Source: CAD feature listing. Evaluate the final solid. Frame: model axes, mm. Face numbers are marked on the shaded views. Give positions to 0.01 mm unless a question says otherwise; leave off trailing zeros. Order: outer loops, then holes, each group sorted by start corner. A loop starts at its lowest first (then second) coordinate and runs counter-clockwise, first axis right, second up. Notation, with made-up numbers: (-9.75, 27.25) -> (20.25, 27.25) arc R10 ccw to (20.25, 41.25) -> close; hole circle Ø5 at (81, -15.5). An arc over 180 degrees is marked (long way). Answer in a Markdown table with one row per item.
```python
from build123d import *

# Parameters (mm, degrees)
SKETCH1_W           = 5.2324
SKETCH1_H           = 13.97
BOSS_EXTRUDE1_DEPTH = 1.524
BOSS_EXTRUDE2_DEPTH = 12.954
SKETCH3_W           = 1.1176
SKETCH3_H           = 1.524
BOSS_EXTRUDE3_DEPTH = 1.016
SKETCH4_W           = 3.81
SKETCH4_H           = 0.1651
BOSS_EXTRUDE4_DEPTH = 1.016
SKETCH5_W           = 3.81
SKETCH5_H           = 0.1651
BOSS_EXTRUDE5_DEPTH = 1.3589
SKETCH6_W           = 13.8049
SKETCH6_H           = 1.3589
CUT_EXTRUDE1_DEPTH  = 0.9525
SKETCH7_W           = 13.8049
SKETCH7_H           = 1.3589
CUT_EXTRUDE2_DEPTH  = 2.4384
SKETCH8_W           = 1.651
SKETCH8_H           = 0.381
CUT_EXTRUDE3_DEPTH  = 1.524
CUT_EXTRUDE4_DEPTH  = 10.995150124
CHAMFER1_SIZE       = 1.143
CHAMFER1_SIZE2      = 0.9906
CHAMFER2_SIZE       = 1.143
CHAMFER2_SIZE_2     = 0.9906


with BuildPart() as part:
    # Sketch1 → Boss-Extrude1 (new body)
    with BuildSketch(Plane(origin=(0, 1.524, 0), x_dir=(-1, 0, 0), z_dir=(0, 1, 0))):
        with Locations((-4.3688, 0)):
            Rectangle(SKETCH1_W, SKETCH1_H)
    extrude(amount=-BOSS_EXTRUDE1_DEPTH)

    # Sketch2 → Boss-Extrude2 (add)
    with BuildSketch(Plane.XY.offset(6.985)):
        Polygon((-5.8674, 1.3589), (1.7526, 1.3589), (1.7526, 1.524), (-6.985, 1.524), (-6.985, 0), (-5.8674, 0), align=None)
    extrude(amount=-BOSS_EXTRUDE2_DEPTH)

    # Sketch3 → Boss-Extrude3 (add)
    with BuildSketch(Plane(origin=(0, 0, -5.969), x_dir=(-1, 0, 0), z_dir=(0, 0, -1))):
        with Locations((6.4262, 0.762)):
            Rectangle(SKETCH3_W, SKETCH3_H)
    extrude(amount=BOSS_EXTRUDE3_DEPTH)

    # Sketch4 → Boss-Extrude4 (add)
    with BuildSketch(Plane(origin=(0, 0, -5.969), x_dir=(-1, 0, 0), z_dir=(0, 0, -1))):
        with Locations((2.0574, 1.44145)):
            Rectangle(SKETCH4_W, SKETCH4_H)
    extrude(amount=BOSS_EXTRUDE4_DEPTH)

    # Sketch5 → Boss-Extrude5 (add)
    with BuildSketch(Plane.XZ.offset(-1.3589)):
        with Locations((-2.0574, -6.90245)):
            Rectangle(SKETCH5_W, SKETCH5_H)
    extrude(amount=BOSS_EXTRUDE5_DEPTH)

    # Sketch6 → Cut-Extrude1 (cut)
    with BuildSketch(Plane(origin=(-5.8674, 0, 0), x_dir=(0, 0, -1), z_dir=(1, 0, 0))):
        with Locations((-0.08255, 0.67945)):
            Rectangle(SKETCH6_W, SKETCH6_H)
    extrude(amount=-CUT_EXTRUDE1_DEPTH, mode=Mode.SUBTRACT)

    # Sketch7 → Cut-Extrude2 (cut)
    with BuildSketch(Plane.ZY.offset(-1.7526)):
        with Locations((0.08255, 0.67945)):
            Rectangle(SKETCH7_W, SKETCH7_H)
    extrude(amount=-CUT_EXTRUDE2_DEPTH, mode=Mode.SUBTRACT)

    # Sketch8 → Cut-Extrude3 (cut)
    with BuildSketch(Plane(origin=(0, 1.524, 0), x_dir=(-1, 0, 0), z_dir=(0, 1, 0))):
        with Locations((-6.1595, -6.7945)):
            Rectangle(SKETCH8_W, SKETCH8_H)
    extrude(amount=-CUT_EXTRUDE3_DEPTH, mode=Mode.SUBTRACT)

    # Sketch9 → Cut-Extrude4 (cut, through all)
    with BuildSketch(Plane(origin=(0, 1.524, 0), x_dir=(-1, 0, 0), z_dir=(0, 1, 0))):
        with BuildLine():
            Line((3.8227, 2.860968655), (3.8227, 5.461))
            Line((3.8227, 5.461), (-0.1143, 5.461))
            Line((-0.1143, 5.461), (-0.1143, 2.860968655))
            ThreePointArc((-0.1143, 2.860968655), (-0.223375415, 2.735239942), (-0.363240303, 2.825478341))
            Line((-0.363240303, 2.825478341), (-1.1303, 5.461))
            Line((-1.1303, 5.461), (-2.3114, 5.461))
            Line((-2.3114, 5.461), (-2.3114, 1.778))
            Line((-2.3114, 1.778), (6.0198, 1.778))
            Line((6.0198, 1.778), (6.0198, 5.461))
            Line((6.0198, 5.461), (4.8387, 5.461))
            Line((4.8387, 5.461), (4.071640303, 2.825478341))
            ThreePointArc((4.071640303, 2.825478341), (3.931775415, 2.735239942), (3.8227, 2.860968655))
        make_face()
    extrude(amount=-CUT_EXTRUDE4_DEPTH, mode=Mode.SUBTRACT)

    # Chamfer1
    chamfer1_edges = [part.edges().sort_by_distance(p)[0] for p in [
        (-6.0198, 1.44145, 1.778),
    ]]
    chamfer1_side = [part.faces().sort_by_distance(p)[0] for p in [
        (-6.0198, 1.44145, 3.6195),
    ]]
    chamfer(chamfer1_edges, length=CHAMFER1_SIZE, length2=CHAMFER1_SIZE2, reference=chamfer1_side[0])

    # Chamfer2
    # the kernel refuses this chamfer: 1.143, 0.9906 mm, written as the material it takes off along each edge
    with BuildSketch(Plane(origin=(2.3114, 1.524, 1.778), x_dir=(0, 0.025420360363461764, -0.9996768504266725), z_dir=(-1, 0, 0))) as chamfer2_piece_1_section:
        Polygon((CHAMFER2_SIZE * 0.999676850427, CHAMFER2_SIZE * 0.0254203603635), (-CHAMFER2_SIZE_2 * 0.0254203603635, CHAMFER2_SIZE_2 * 0.999676850427), (0, 0), align=None)
    chamfer2_piece_1 = extrude(amount=10.285426882, mode=Mode.PRIVATE)
    chamfer2_piece_1 = split(chamfer2_piece_1, bisect_by=Plane(origin=(-3.105218089, 1.443787017, -0.441979128), z_dir=(0.7556890827898172, 0, 0.6549305384178423)), keep=Keep.TOP, mode=Mode.PRIVATE)
    add(chamfer2_piece_1, mode=Mode.SUBTRACT)


solid = part.part
```
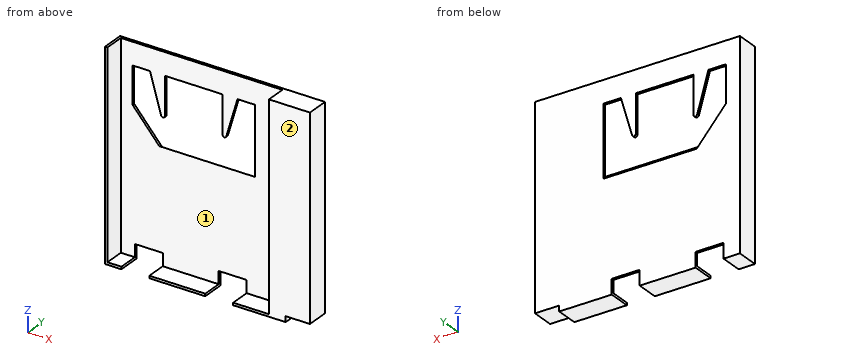
(1) Section query D-D (z = 5). Return the cut outline in (x, y) (3 decimals), plus the area to 3 significant figures.
A:
| item | result |
|---|---|
| outline | (-6.985, 0) -> (-6.82, 0) -> (-6.82, 1.359) -> (-6.02, 1.359) -> (-6.02, 1.524) -> (-6.985, 1.524) -> close; (-4.705, 1.359) -> (-3.823, 1.359) -> (-3.823, 1.524) -> (-4.705, 1.524) -> close; (0.114, 1.359) -> (0.996, 1.359) -> (0.996, 1.524) -> (0.114, 1.524) -> close; (2.311, 1.359) -> (4.191, 1.359) -> (4.191, 0) -> (6.985, 0) -> (6.985, 1.524) -> (2.311, 1.524) -> close |
| area | 5.24 mm^2 |
(2) Ray query, probe 1 along X at (y, z) = (0.7, 0) (3 decimals); probe 2 along X at (y, z) = (1.4, 5.25) (3 decimals); probe 3 along Z at (x, y) = (-0.5, 1.2) (3 decimals). Return the intervals inside material, ascending.
A:
| item | result |
|---|---|
| probe 1 | x = -6.985 to -6.82, 4.191 to 6.985 |
| probe 2 | x = -6.985 to -6.02, -4.777 to -3.823, 0.114 to 1.069, 2.311 to 6.985 |
| probe 3 | z = -6.985 to -6.82 |
(3) Section query B-B (y = 0.9). Return the cut outline in (x, z) (3 decimals), plus the area to 3 significant figures.
A:
| item | result |
|---|---|
| outline | (-6.985, -6.985) -> (-5.867, -6.985) -> (-5.867, -6.82) -> (-6.82, -6.82) -> (-6.82, 6.985) -> (-6.985, 6.985) -> close; (-3.962, -6.985) -> (-0.152, -6.985) -> (-0.152, -6.82) -> (-3.962, -6.82) -> close; (1.753, -6.985) -> (5.334, -6.985) -> (5.334, -6.604) -> (6.985, -6.604) -> (6.985, 6.985) -> (4.191, 6.985) -> (4.191, -6.82) -> (1.753, -6.82) -> close |
| area | 41.9 mm^2 |
(4) First-contact query: pin 1 Ø6 at (x, z) = (5, -1.5) entering from -Y. Flat tip, straight axial feed; report the tip coordinate or a pass-through.
A:
| item | result |
|---|---|
| pin 1 | stops at y = 0 |
(5) Section query C-C (z = 1.5). Return the cut outline in (x, y) (3 decimals), plus the area to 3 significant figures.
A:
| item | result |
|---|---|
| outline | (-6.985, 0) -> (-6.82, 0) -> (-6.82, 1.359) -> (-4.788, 1.359) -> (-4.788, 1.524) -> (-6.985, 1.524) -> close; (2.311, 1.359) -> (4.191, 1.359) -> (4.191, 0) -> (6.985, 0) -> (6.985, 1.524) -> (2.311, 1.524) -> close |
| area | 5.16 mm^2 |
(6) Pull-direction query (X, two-part tool) for the marked faces 1 and 2; classes: +X half, -X half, draft (parallel to the pull), parting line (faces both ways), or undercut.
A:
| item | result |
|---|---|
| face 1 | undercut |
| face 2 | draft |
